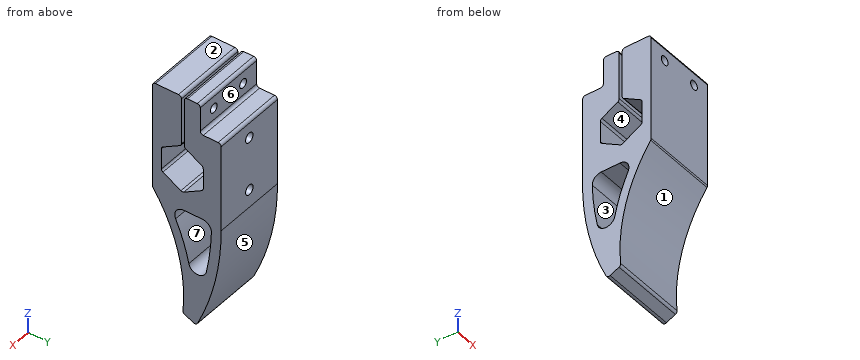
```python
from build123d import *

# Parameters (mm, degrees)
BOSS_EXTRUDE1_DEPTH   = 25
FILLET1_R             = 1
F_3_0MM_DOWEL_HOLE1_D = 3
M4_TAPPED_HOLE1_D     = 3.3
M4_TAPPED_HOLE1_DEPTH = 10.1
M4_TAPPED_HOLE1_TIP   = 0.991420021


with BuildPart() as part:
    # Sketch1 → Boss-Extrude1 (new body)
    with BuildSketch(Plane(origin=(0, 0, 0), x_dir=(0, 0, -1), z_dir=(1, 0, 0))):
        with BuildLine():
            Line((0, 85), (-30, 85))
            Line((-30, 85), (-30, 78))
            Line((-30, 78), (-40, 78))
            Line((-40, 78), (-40, 72.7))
            Line((-40, 72.7), (-22.67875858, 72.7))
            Line((-22.67875858, 72.7), (-19.041451884, 79))
            Line((-19.041451884, 79), (-10.958548116, 79))
            Line((-10.958548116, 79), (-6.917096231, 72))
            Line((-6.917096231, 72), (-10.958548116, 65))
            Line((-10.958548116, 65), (-19.041451884, 65))
            Line((-19.041451884, 65), (-22.909698688, 71.7))
            Line((-22.909698688, 71.7), (-40, 71.7))
            Line((-40, 71.7), (-40, 62))
            Line((-40, 62), (-4, 62))
            ThreePointArc((-4, 62), (14.367926682, 70.556066939), (34.568411175, 72.145858848))
            Line((34.568411175, 72.145858848), (36.728936873, 76.654975026))
            ThreePointArc((36.728936873, 76.654975026), (18.832513412, 82.887492655), (0, 85))
        make_face()
        with BuildLine():
            Line((-0.917096231, 72.45580085), (-0.917096231, 78.731121633))
            ThreePointArc((-0.917096231, 78.731121633), (-0.009883557, 80.880596268), (2.163064575, 81.730050482))
            ThreePointArc((2.163064575, 81.730050482), (9.436412465, 81.210823112), (16.634722164, 80.046553355))
            ThreePointArc((16.634722164, 80.046553355), (19.024323748, 77.110478101), (16.637014487, 74.172538667))
            ThreePointArc((16.637014487, 74.172538667), (9.867798138, 72.343342951), (3.357045186, 69.739817851))
            ThreePointArc((3.357045186, 69.739817851), (0.473932708, 69.9237637), (-0.917096231, 72.45580085))
        make_face(mode=Mode.SUBTRACT)
    extrude(amount=BOSS_EXTRUDE1_DEPTH)

    # Fillet1
    fillet1_edges = [part.edges().sort_by_distance(p)[0] for p in [
        (12.5, 76.654975026, -36.728936873),
        (12.5, 72.145858848, -34.568411175),
        (12.5, 62, 4),
        (12.5, 62, 40),
        (12.5, 71.7, 40),
        (12.5, 71.7, 22.909698688),
        (12.5, 65, 19.041451884),
        (12.5, 65, 10.958548116),
        (12.5, 72, 6.917096231),
        (12.5, 79, 10.958548116),
        (12.5, 79, 19.041451884),
        (12.5, 72.7, 22.67875858),
        (12.5, 72.7, 40),
        (12.5, 78, 40),
        (12.5, 78, 30),
        (12.5, 85, 30),
    ]]
    fillet(fillet1_edges, radius=FILLET1_R)

    # Ø3.0mm Dowel Hole1 (through all)
    with Locations(Plane(origin=(0, 78, 0), x_dir=(1, 0, 0), z_dir=(0, 1, 0))):
        with Locations((6, -35), (19, -35)):
            Hole(F_3_0MM_DOWEL_HOLE1_D / 2)

    # M4 Tapped Hole1
    with Locations(Plane(origin=(0, 85, 0), x_dir=(1, 0, 0), z_dir=(0, 1, 0))):
        with Locations((12.5, -24), (12.5, -6)):
            Hole(M4_TAPPED_HOLE1_D / 2, depth=M4_TAPPED_HOLE1_DEPTH)
            with Locations((0, 0, -(M4_TAPPED_HOLE1_DEPTH + M4_TAPPED_HOLE1_TIP / 2))):  # 118° drill point
                Cone(0, M4_TAPPED_HOLE1_D / 2, M4_TAPPED_HOLE1_TIP, mode=Mode.SUBTRACT)


solid = part.part
```
The model under review builds one solid part; all positions refer to its coordinate system, in mm. Face numbers are marked on the shaded views. A direction names the side the tool comes from. Round coordinates to 2 decimals unless told otherwise and drop trailing zeros. Write each loop counter-clockwise with the first axis right and the second up, starting at its lowest first coordinate (ties: lowest second). Pieces come first, ordered by that corner, then holes. Notation, with made-up numbers: (-34, -15.75) - (10, -15.75) arc R10 cw to (10, -9.75) - close; hole circle Ø11 at (3.25, 11.25). An arc over 180 degrees is marked (long way). Use one line per item in the form item = value.
Q1. Tool access review of the marked faces 5, 6 and 7: name each direction out of +Z, -Z, +X, -X, +Y, -Y from which nothing blocks a thin tool from reaching the whole face with its end or side.
Answer key:
face_5 = -Z, +X, -X, +Y
face_6 = +Z, +X, -X, +Y
face_7 = +X, -X
Q2. For line 1 (X direction, y = 66.25, z = 35); line 2 (Z direction, x = 19, y = 75.35); line 3 (Y direction, x = 8.75, z = 31.5), list the stretches that pass through material, from the lowest coordinate up. Write a range as [from, to].
Answer key:
line_1 = [0, 4.5], [7.5, 17.5], [20.5, 25]
line_2 = [-36.1, -18.45], [0.92, 8.85], [21.15, 33.5], [36.5, 40]
line_3 = [62, 71.7], [72.7, 78]
Q3. Consider section C-C (y = 80.75). State the section outline as (x, z) points, and give its area (3 significant figures).
Answer key:
outline = (0, -26.54) - (25, -26.54) - (25, -12.79) - (0, -12.79) - close; (0, 0.14) - (25, 0.14) - (25, 30) - (0, 30) - close; hole circle Ø3.3 at (12.5, 6); hole circle Ø3.3 at (12.5, 24)
area = 1,070 mm2
Q4. Draft analysis for pull direction Y (two halves, no side actions). For the marked faces 1, 2, 3 and 4, state which applies: +Y half, -Y half, draft (parallel to the pull), parting line (faces both ways), or undercut.
Answer key:
face_1 = -Y half
face_2 = draft
face_3 = undercut
face_4 = undercut
Q5. Consider section D-D (x = 6). State how many separate pieces and enclosed holes the cut face has, and give its area (3 significant figures).
Answer key:
separate_pieces = 3
enclosed_holes = 1
area = 867 mm2
Q6. Insertion check: pin 1 Ø4 at (x, z) = (19, 35) entering from +Y; pin 2 Ø8 at (x, z) = (9.5, -20.5) entering from +Y; pin 3 Ø2.5 at (x, y) = (11.5, 82) entering from +Z; pin 4 Ø8 at (y, z) = (67, -28.5) entering from -X. Each pin has a flat end and moves straight along its axis. Give the tip position at first contact, or say it passes through.
Answer key:
pin_1 = 78
pin_2 = 83.38
pin_3 = 30
pin_4 = through
Q7. Consider section A-A (z = 35). State the section outline as (x, y) points, and give its area (3 significant figures).
Answer key:
outline = (0, 62) - (4.5, 62) - (4.5, 71.7) - (0, 71.7) - close; (0, 72.7) - (4.5, 72.7) - (4.5, 78) - (0, 78) - close; (7.5, 62) - (17.5, 62) - (17.5, 71.7) - (7.5, 71.7) - close; (7.5, 72.7) - (17.5, 72.7) - (17.5, 78) - (7.5, 78) - close; (20.5, 62) - (25, 62) - (25, 71.7) - (20.5, 71.7) - close; (20.5, 72.7) - (25, 72.7) - (25, 78) - (20.5, 78) - close
area = 285 mm2
Q8. Consider section B-B (z = 14). State the section outline as (x, y) points, and give its area (3 significant figures).
Answer key:
outline = (0, 62) - (25, 62) - (25, 65) - (0, 65) - close; (0, 79) - (25, 79) - (25, 85) - (0, 85) - close
area = 225 mm2
